The listing builds one solid part. Answer for the finished solid, in the listing's coordinates (mm). A direction names the side the tool comes from. Give positions to 0.01 mm unless a question says otherwise; leave off trailing zeros. Order: outer loops, then holes, each group sorted by start corner. A loop starts at its lowest first (then second) coordinate and runs counter-clockwise, first axis right, second up. Notation, with made-up numbers: (-15, 42) - (-10, 42) arc R8 ccw to (-10, 48) - close; hole circle Ø3 at (-22, 36.5). An arc over 180 degrees is marked (long way). Answer as CSV lines item,"result". Start each with the question number.
1. Flat-ended cylindrical pins translate along their axes: pin 1 (0.5 mm diameter, centred on x = 0.5, y = 0, fed in from +Z); pin 2 (1.5 mm diameter, centred on x = 29, y = -1, fed in from -Z). Find the tip coordinate at first contact, or state that the pin passes through.
2. Consider line 1 along Z through (x, y) = (7, -0.45); line 2 along X through (y, z) = (-0.5, -0.4); line 3 along Y through (x, z) = (7, 0). Determine where each line is inside the solid, lowest interval first. Write a range as [from, to].
3. Which of the six approach directions +Z, -Z, +X, -X, +Y, -Y give full straight-line access (tool end or side, diameter ignored) to faces 5 (the flat face through (1.6, -2, 1)), 6 (the flat face through (0.5, 0, -1)), 7 (the cylindrical face through (1.427, 2.337, 0.969))?
4. Section A-A on x = 18.5 is taken. Give the vertices of the cut face in (y, z), and give its area (3 significant figures).
5. Determine the mould class of faces 1 (the flat face through (1, 0, 0)), 2 (the cylindrical face through (20.53, -1.5, -0.07)), 3 (the flat face through (0.49, -0.86, -0.51)), 4 (the flat face through (38.6, 0, 0)) for opening direction Y: +Y half, -Y half, draft (parallel to the pull), parting line (faces both ways), or undercut.
from build123d import *

# Parameters (mm, degrees)
CUT_EXTRUDE1_DEPTH = 1


with BuildPart() as part:
    # Sketch2 → Revolve1 (revolve)
    with BuildSketch(Plane.XY):
        with BuildLine():
            Line((0, 0), (0, 1.43))
            ThreePointArc((0, 1.43), (0.558633593, 2.055416372), (1.25, 2.53))
            Line((1.25, 2.53), (1.6, 2.53))
            Line((1.6, 2.53), (1.6, 1.85))
            Line((1.6, 1.85), (1.95, 1.5))
            Line((1.95, 1.5), (38.6, 1.5))
            Line((38.6, 1.5), (38.6, 0))
            Line((38.6, 0), (0, 0))
        make_face()
    revolve(axis=Axis((38.6, 0, 0), (-1, 0, 0)))

    # Sketch3 → Cut-Extrude1 (cut)
    with BuildSketch(Plane.ZY):
        Polygon((0, 1.154700538), (-1, 0.577350269), (-1, -0.577350269), (0, -1.154700538), (1, -0.577350269), (1, 0.577350269), align=None)
    extrude(amount=-CUT_EXTRUDE1_DEPTH, mode=Mode.SUBTRACT)


solid = part.part
Checks:
1,pin 1,"stops at z = 2.21"
1,pin 2,"stops at z = -1.48"
2,line 1,"z = [-1.43, 1.43]"
2,line 2,"x = [1, 38.6]"
2,line 3,"y = [-1.5, 1.5]"
3,face 5,"+X"
3,face 6,"-X"
3,face 7,"+X, -X"
4,outline,"circle Ø3 at (0, 0)"
4,area,"7.07 mm²"
5,face 1,"undercut"
5,face 2,"parting line"
5,face 3,"undercut"
5,face 4,"draft"
